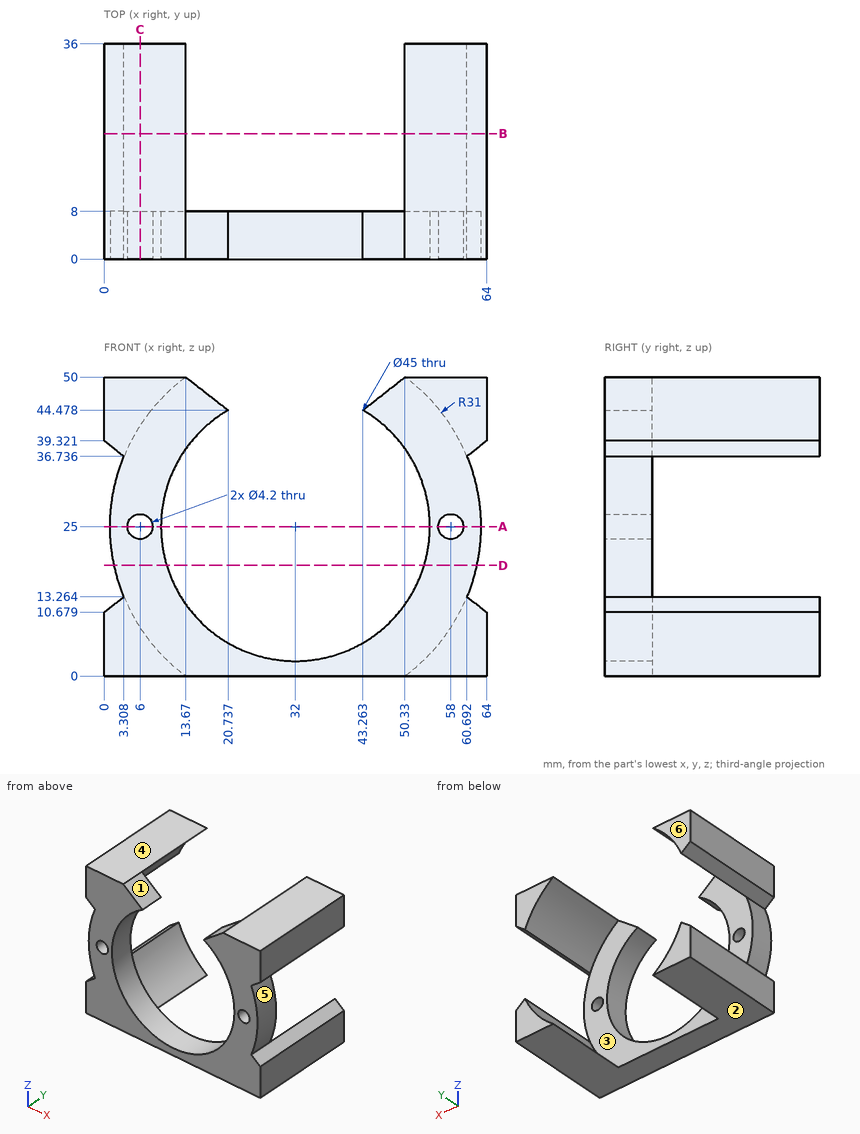
Study the drawing (mm; zero at the part's minimum x, y, z) and answer. A direction names the side the tool comes from. Coordinates: 2 decimals unless noted, no trailing zeros. Loops run counter-clockwise (first coordinate to the right, second up) from the corner with the lowest first, then second, coordinate; pieces in that order, holes last. Notation, with made-up numbers: (19.5, 19.25) -> (55.5, 19.25) arc R10 ccw to (55.5, 30.25) -> close; hole circle Ø9 at (19, -21). An arc over 180 degrees is marked (long way). Answer in a Markdown table with one row per item. Add a question column.
1. Flat-ended cylindrical pins translate along their axes: P1, Ø3, axis at y = 17.5, z = 36, coming from the +X side; P2, Ø5, axis at x = 55.5, y = 23, coming from the -Z side; P3, Ø1.5, axis at y = 14.5, z = 11.5, coming from the -X side; P4, Ø1.5, axis at y = 7, z = 14.5, coming from the -X side. Find the tip coordinate at first contact, or state that the pin passes through.
2. The part is cut by section A-A, the plane z = 25. Write down the section's boundary in (x, y).
3. For the marked faces 1, 2 and 3, determine the directions among +Z, -Z, +X, -X, +Y, -Y from which every point of the face is accessible in a straight line to the end or side of a thin tool.
4. Determine the mould class of the marked faces 4, 5 and 6 for opening direction Z: +Z half, -Z half, draft (parallel to the pull), parting line (faces both ways), or undercut.
5. The part is cut by section B-B, the plane y = 21. Write down the section's boundary in (x, z) (1 decimal).
6. Consider line 1 (X direction, y = 4, z = 25); line 2 (Y direction, x = 11, z = 36); line 3 (Z direction, x = 46, y = 3.5) (1 decimal). Determine where each line is inside the solid, lowest interval first. Write a range as [from, to].
7. The part is cut by section C-C, the plane x = 6. Write down the section's boundary in (y, z).
8. The part is cut by section D-D, the plane z = 18.5. Write down the section's boundary in (x, y), then the cut area to 3 significant figures.
Answer below:
| question | item | result |
|---|---|---|
| 1 | P1 | x = 61.67 |
| 1 | P2 | z = 0 |
| 1 | P3 | x = 0.09 |
| 1 | P4 | x = 2.57 |
| 2 | outline | (1, 0) -> (3.9, 0) -> (3.9, 8) -> (1, 8) -> close; (8.1, 0) -> (9.5, 0) -> (9.5, 8) -> (8.1, 8) -> close; (54.5, 0) -> (55.9, 0) -> (55.9, 8) -> (54.5, 8) -> close; (60.1, 0) -> (63, 0) -> (63, 8) -> (60.1, 8) -> close |
| 3 | face 1 | +Z, +Y, -Y |
| 3 | face 2 | -Z, +X, -X, +Y, -Y |
| 3 | face 3 | +Y |
| 4 | face 4 | +Z half |
| 4 | face 5 | undercut |
| 4 | face 6 | draft |
| 5 | outline | (0, 0) -> (13.7, 0) arc R31 cw to (3.3, 13.3) -> (0, 10.7) -> close; (0, 39.3) -> (3.3, 36.7) arc R31 cw to (13.7, 50) -> (0, 50) -> close; (50.3, 0) -> (64, 0) -> (64, 10.7) -> (60.7, 13.3) arc R31 cw to start; (50.3, 50) arc R31 cw to (60.7, 36.7) -> (64, 39.3) -> (64, 50) -> close |
| 6 | line 1 | [1, 3.9], [8.1, 9.5], [54.5, 55.9], [60.1, 63] |
| 6 | line 2 | [0, 8] |
| 6 | line 3 | [0, 7.4], [42.6, 46.6] |
| 7 | outline | (0, 0) -> (36, 0) -> (36, 8.12) -> (8, 8.12) -> (8, 22.9) -> (0, 22.9) -> close; (0, 27.1) -> (8, 27.1) -> (8, 41.88) -> (36, 41.88) -> (36, 50) -> (0, 50) -> close |
| 8 | outline | (1.69, 0) -> (10.46, 0) -> (10.46, 8) -> (1.69, 8) -> close; (53.54, 0) -> (62.31, 0) -> (62.31, 8) -> (53.54, 8) -> close |
| 8 | area | 140 mm2 |
